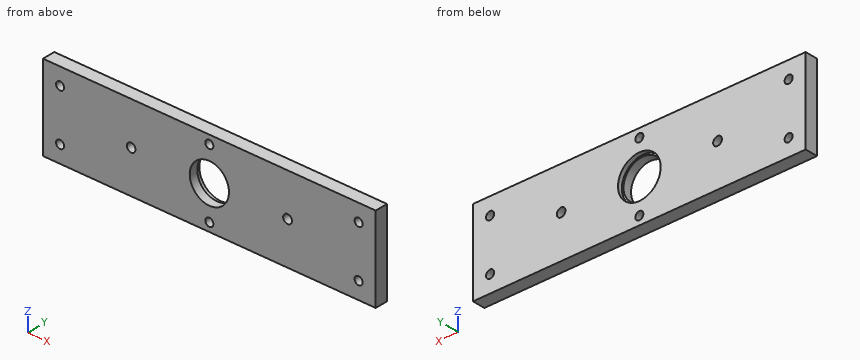
```python
from build123d import *

# Parameters (mm, degrees)
SKETCH1_W                  = 247.65
SKETCH1_H                  = 63.5
BOSS_EXTRUDE1_DEPTH        = 9.525
SKETCH3_R                  = 14.605
CUT_EXTRUDE1_DEPTH         = 129.185095662
F_6_0_6_DIAMETER_HOLE1_D   = 6
F_6_5_6_5_DIAMETER_HOLE3_D = 6.5
SKETCH29_R                 = 15.875
CUT_EXTRUDE5_DEPTH         = 3.175
F_6_0_6_DIAMETER_HOLE3_D   = 6


with BuildPart() as part:
    # Sketch1 → Boss-Extrude1 (new body)
    with BuildSketch(Plane(origin=(0, 0, 0), x_dir=(1, 0, 0), z_dir=(0, 1, 0))):
        Rectangle(SKETCH1_W, SKETCH1_H)
    extrude(amount=BOSS_EXTRUDE1_DEPTH)

    # Sketch3 → Cut-Extrude1 (cut, through all)
    with BuildSketch(Plane(origin=(0, 9.525, 0), x_dir=(1, 0, 0), z_dir=(0, 1, 0))):
        with Locations(Location((0, 0, 0), (0, 0, 270))):
            Circle(SKETCH3_R)
    extrude(amount=-CUT_EXTRUDE1_DEPTH, mode=Mode.SUBTRACT)

    # Ø6.0 (6) Diameter Hole1 (through all)
    with Locations(Plane(origin=(0, 0, 0), x_dir=(-1, 0, 0), z_dir=(0, -1, 0))):
        with Locations((0, -25.4), (0, 25.4)):
            Hole(F_6_0_6_DIAMETER_HOLE1_D / 2)

    # Ø6.5 (6.5) Diameter Hole3 (through all)
    with Locations(Plane(origin=(0, 0, 0), x_dir=(-1, 0, 0), z_dir=(0, -1, 0))):
        with Locations((58.208333333, 0), (-58.208333333, 0)):
            Hole(F_6_5_6_5_DIAMETER_HOLE3_D / 2)

    # Sketch29 → Cut-Extrude5 (cut)
    with BuildSketch(Plane(origin=(0, 9.525, 0), x_dir=(1, 0, 0), z_dir=(0, 1, 0))):
        with Locations(Location((0, 0, 0), (0, 0, 270))):
            Circle(SKETCH29_R)
    extrude(amount=-CUT_EXTRUDE5_DEPTH, mode=Mode.SUBTRACT)

    # Ø6.0 (6) Diameter Hole3 (through all)
    with Locations(Plane(origin=(0, 9.525, 0), x_dir=(1, 0, 0), z_dir=(0, 1, 0))):
        with Locations((-111.125, 19.05), (-111.125, -19.05), (111.125, -19.05), (111.125, 19.05)):
            Hole(F_6_0_6_DIAMETER_HOLE3_D / 2)


solid = part.part
```
Verification items for the finished model (mm, model axes). Round coordinates to 2 decimals unless told otherwise and drop trailing zeros. Write each loop counter-clockwise with the first axis right and the second up, starting at its lowest first coordinate (ties: lowest second). Pieces come first, ordered by that corner, then holes. Notation, with made-up numbers: (65.5, -7.75) - (93.5, -7.75) arc R21 ccw to (93.5, 26.25) - close; hole circle Ø8 at (-4, -36). An arc over 180 degrees is marked (long way). Answer as a JSON object with one key per item and string values. Group by question number.
Q1. Section check D-D, the plane z = 9. Enter the section's corners in (x, y) (3 decimals).
Q2. Go/stop test with a flat-tipped pin: pin 1 Ø3.5 at (x, z) = (111.125, 19.05) entering from -Y. Record where the tip stops, or that it passes through.
Q3. Thickness scan on line 1 (X direction, y = 2.75, z = -19.05) (3 decimals); line 2 (X direction, y = 9, z = -25.5) (3 decimals); line 3 (X direction, y = 3, z = -3) (3 decimals). Record the ranges inside material, lowest first.
Q4. Section check B-B, the plane y = 8. Give the number of separate pieces and of enclosed holes in the cut face, plus the area to 3 significant figures.
Q5. Section check C-C, the plane z = 0. Enter the section's corners in (x, y) (3 decimals).
Q6. Section check A-A, the plane z = 25.4. Enter the section's corners in (x, y) (3 decimals), plus the area to 3 significant figures.
Found:
{
 "1": {"outline": "(-123.825, 0) - (-11.502, 0) - (-11.502, 6.35) - (-13.077, 6.35) - (-13.077, 9.525) - (-123.825, 9.525) - close; (11.502, 0) - (123.825, 0) - (123.825, 9.525) - (13.077, 9.525) - (13.077, 6.35) - (11.502, 6.35) - close"},
 "2": {"pin 1": "passes through"},
 "3": {"line 1": "x = -123.825 to -114.125, -108.125 to 108.125, 114.125 to 123.825", "line 2": "x = -123.825 to -2.998, 2.998 to 123.825", "line 3": "x = -123.825 to -59.458, -56.958 to -14.294, 14.294 to 56.958, 59.458 to 123.825"},
 "4": {"separate pieces": "1", "enclosed holes": "9", "area": "14,700 mm^2"},
 "5": {"outline": "(-123.825, 0) - (-61.458, 0) - (-61.458, 9.525) - (-123.825, 9.525) - close; (-54.958, 0) - (-14.605, 0) - (-14.605, 6.35) - (-15.875, 6.35) - (-15.875, 9.525) - (-54.958, 9.525) - close; (14.605, 0) - (54.958, 0) - (54.958, 9.525) - (15.875, 9.525) - (15.875, 6.35) - (14.605, 6.35) - close; (61.458, 0) - (123.825, 0) - (123.825, 9.525) - (61.458, 9.525) - close"},
 "6": {"outline": "(-123.825, 0) - (-3, 0) - (-3, 9.525) - (-123.825, 9.525) - close; (3, 0) - (123.825, 0) - (123.825, 9.525) - (3, 9.525) - close", "area": "2,300 mm^2"}
}
